Part model, mm, in its own coordinate system. Face numbers are marked on the shaded views. Round coordinates to 2 decimals unless told otherwise and drop trailing zeros. Loops run counter-clockwise (first coordinate to the right, second up) from the corner with the lowest first, then second, coordinate; pieces in that order, holes last.
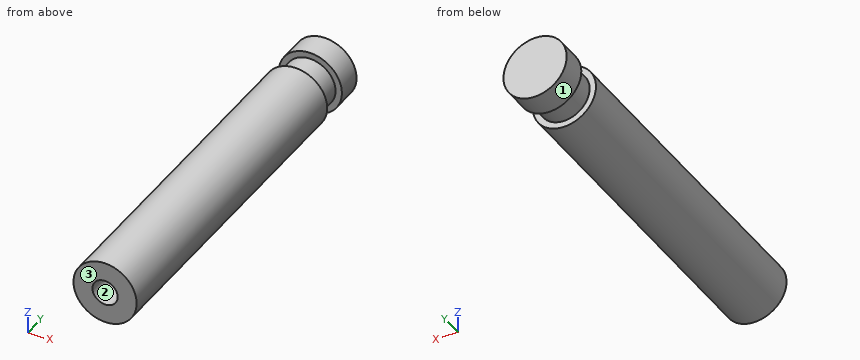
from build123d import *

# Parameters (mm, degrees)
SKETCH1_R           = 2.5
BOSS_EXTRUDE1_DEPTH = 26
SKETCH1_5_R         = 1
CUT_EXTRUDE1_DEPTH  = 10
SKETCH3_R           = 2
BOSS_EXTRUDE2_DEPTH = 2
SKETCH4_R           = 2.5
BOSS_EXTRUDE3_DEPTH = 2


with BuildPart() as part:
    # Sketch1 → Boss-Extrude1 (new body)
    with BuildSketch(Plane(origin=(0, 0, 0), x_dir=(1, 0, 0), z_dir=(0, 1, 0))):
        with Locations(Location((0, 0, 0), (0, 0, 270))):
            Circle(SKETCH1_R)
    extrude(amount=BOSS_EXTRUDE1_DEPTH)

    # Sketch1_5 → Cut-Extrude1 (cut)
    with BuildSketch(Plane(origin=(0, 0, 0), x_dir=(1, 0, 0), z_dir=(0, 1, 0))):
        with Locations(Location((0, 0, 0), (0, 0, 270))):
            Circle(SKETCH1_5_R)
    extrude(amount=CUT_EXTRUDE1_DEPTH, mode=Mode.SUBTRACT)

    # Sketch3 → Boss-Extrude2 (add)
    with BuildSketch(Plane(origin=(0, 26, 0), x_dir=(1, 0, 0), z_dir=(0, 1, 0))):
        with Locations(Location((0, 0, 0), (0, 0, 270))):
            Circle(SKETCH3_R)
    extrude(amount=BOSS_EXTRUDE2_DEPTH)

    # Sketch4 → Boss-Extrude3 (add)
    with BuildSketch(Plane(origin=(0, 28, 0), x_dir=(1, 0, 0), z_dir=(0, 1, 0))):
        with Locations(Location((0, 0, 0), (0, 0, 270))):
            Circle(SKETCH4_R)
    extrude(amount=BOSS_EXTRUDE3_DEPTH)


solid = part.part
1) Slice it at C-C, the plane y = 6. Give the cut face in (x, z).
Values:
outline: circle Ø5 at (0, 0); hole circle Ø2 at (0, 0)
2) Mould opens along Z. For the marked faces 1, 2 and 3 say: released by +Z, released by -Z, zero draft, split by the parting line, or undercut.
Values:
face 1: split by the parting line
face 2: undercut
face 3: zero draft
3) Slice it at A-A, the plane z = 0. Give the cut face in (x, y).
Values:
outline: (-2.5, 0) - (-1, 0) - (-1, 10) - (1, 10) - (1, 0) - (2.5, 0) - (2.5, 26) - (2, 26) - (2, 28) - (2.5, 28) - (2.5, 30) - (-2.5, 30) - (-2.5, 28) - (-2, 28) - (-2, 26) - (-2.5, 26) - close
4) Drop flat-ended pins along their axis: pin 1 Ø1 at (y, z) = (3.5, 1.5) entering from -X; pin 2 Ø1 at (x, y) = (-1, 21.5) entering from -Z; pin 3 Ø1.5 at (x, y) = (0.5, 27) entering from -Z. Give the stop position or say it passes through.
Values:
pin 1: stops at x = -2.29
pin 2: stops at z = -2.45
pin 3: stops at z = -2
5) Slice it at D-D, the plane y = 17.75. Give the cut face in (x, z), then the cut area to 3 significant figures.
Values:
outline: circle Ø5 at (0, 0)
area: 19.6 mm2
6) Wall check: line 1 along X through (y, z) = (5.25, 0); line 2 along Y through (x, z) = (2.1, 0.6); line 3 along Z through (x, y) = (0.1, 22). Give the ranges that are in metal, low to high.
Values:
line 1: x = -2.5 to -1, 1 to 2.5
line 2: y = 0 to 26, 28 to 30
line 3: z = -2.5 to 2.5
7) Slice it at B-B, the plane x = 0. Give the cut face in (y, z).
Values:
outline: (0, -2.5) - (26, -2.5) - (26, -2) - (28, -2) - (28, -2.5) - (30, -2.5) - (30, 2.5) - (28, 2.5) - (28, 2) - (26, 2) - (26, 2.5) - (0, 2.5) - (0, 1) - (10, 1) - (10, -1) - (0, -1) - close
